The listing builds one solid part. Answer for the finished solid, in the listing's coordinates (mm). A direction names the side the tool comes from. Coordinates: 2 decimals unless noted, no trailing zeros. Loops run counter-clockwise (first coordinate to the right, second up) from the corner with the lowest first, then second, coordinate; pieces in that order, holes last. Notation, with made-up numbers: M -34.75,39 L -10.75,39 A20 ccw -10.75,78 Z; hole C -37.75,65.25 d1. An arc over 180 degrees is marked long. Answer as a JSON object with one key per item and string values. Group by question number.
1. A cutting plane is placed at A-A on y = 22. Give the vertices of the cut face in (x, z), and give its area (3 significant figures).
2. Given pin 1 (2 mm diameter, centred on x = 0, z = -4, fed in from +Y); pin 2 (1.5 mm diameter, centred on x = -2, z = -8.5, fed in from -Y), each flat-ended and moving along its own axis, determine where each tip first touches the part or whether it passes through.
3. For faces 1 (the face through (0, 19.05, -4)), 2 (the face through (-6.35, 13, -6)), determine the directions among +Z, -Z, +X, -X, +Y, -Y from which every point of the face is accessible in a straight line to the end or side of a thin tool.
4. Straight lines are drawn through the part: L1, parallel to Y at x = 0, z = -2.25; L2, parallel to Y at x = 0, z = -1.25; L3, parallel to Z at x = -0.75, y = 1.5. For each, find the intervals that lie inside material, in ascending order.
5. Determine the mould class of faces 3 (the face through (0, 0, -6.35)), 4 (the face through (3.804, 1.198, -3.131)), 5 (the face through (0, 25.4, -6)), 6 (the face through (0, 10, -12.7)) for opening direction Y: released by +Y, released by -Y, zero draft, split by the parting line, or undercut.
from build123d import *

# Parameters (mm, degrees)
SKETCH1_W           = 12.7
SKETCH1_H           = 19.05
SKETCH1_H_2         = 12.7
SKETCH1_R           = 3.9878
BOSS_EXTRUDE1_DEPTH = 12.7
FILLET1_SIZE        = 7.9756
CUT_EXTRUDE2_DEPTH  = 6.35
SKETCH1_3_R         = 3.9878
CUT_EXTRUDE3_DEPTH  = 6.35


with BuildPart() as part:
    # Sketch1 → Boss-Extrude1 (new body)
    # profile 1 of 3: a face of its own
    with BuildSketch(Plane.XY):
        with Locations((0, 15.875)):
            Rectangle(SKETCH1_W, SKETCH1_H)
    # profile 2 of 3: a face of its own
    with BuildSketch(Plane.XY):
        Rectangle(SKETCH1_W, SKETCH1_H_2)
        Circle(SKETCH1_R, mode=Mode.SUBTRACT)
    # profile 3 of 3: a face of its own
    with BuildSketch(Plane.XY):
        Circle(SKETCH1_R)
    extrude(amount=-BOSS_EXTRUDE1_DEPTH)

    # Fillet1
    # a fillet whose section is not a circle: 7.9756 mm, written as the material it takes off along each edge
    with BuildSketch(Plane(origin=(-6.35, -6.35, 19.939), x_dir=(1, 0, 0), z_dir=(0, 0, -1)), Plane(origin=(6.35, -6.35, 19.939), x_dir=(0, 1, 0), z_dir=(0, 0, -1))) as fillet1_piece_1:
        with BuildLine():
            add(Edge.make_bspline([(FILLET1_SIZE, 0), (FILLET1_SIZE * 0.831801948466, 0), (FILLET1_SIZE * 0.663603896932, 0), (FILLET1_SIZE * 0.292893218813, -FILLET1_SIZE * 0.0716919198361), (FILLET1_SIZE * 0.0716919198361, -FILLET1_SIZE * 0.292893218813), (0, -FILLET1_SIZE * 0.663603896932), (0, -FILLET1_SIZE * 0.831801948466), (0, -FILLET1_SIZE)], knots=[0, 0, 0, 0, 0, 0, 0.5, 0.5, 1, 1, 1, 1, 1, 1], degree=5))
            Line((0, -FILLET1_SIZE), (0, 0))
            Line((0, 0), (FILLET1_SIZE, 0))
        make_face()
    extrude(amount=52.578, mode=Mode.SUBTRACT)

    # Sketch3 → Cut-Extrude2 (cut)
    with BuildSketch(Plane(origin=(0, 25.4, 0), x_dir=(1, 0, 0), z_dir=(0, 1, 0))):
        with BuildLine():
            ThreePointArc((1.9939, 8.89), (1.409900211, 10.299900211), (0, 10.8839))
            Line((0, 10.8839), (0, 8.89))
            Line((0, 8.89), (1.9939, 8.89))
        make_face()
        with BuildLine():
            Line((0, 8.89), (0, 10.8839))
            ThreePointArc((0, 10.8839), (-1.409900211, 10.299900211), (-1.9939, 8.89))
            Line((-1.9939, 8.89), (0, 8.89))
        make_face()
        with BuildLine():
            Line((1.9939, 8.89), (0, 8.89))
            Line((0, 8.89), (0, 6.8961))
            ThreePointArc((0, 6.8961), (1.409900211, 7.480099789), (1.9939, 8.89))
        make_face()
        with BuildLine():
            Line((0, 6.8961), (0, 8.89))
            Line((0, 8.89), (-1.9939, 8.89))
            ThreePointArc((-1.9939, 8.89), (-1.409900211, 7.480099789), (0, 6.8961))
        make_face()
        with BuildLine():
            ThreePointArc((1.9939, 3.81), (1.409900211, 5.219900211), (0, 5.8039))
            Line((0, 5.8039), (0, 3.81))
            Line((0, 3.81), (1.9939, 3.81))
        make_face()
        with BuildLine():
            Line((0, 3.81), (0, 5.8039))
            ThreePointArc((0, 5.8039), (-1.409900211, 5.219900211), (-1.9939, 3.81))
            Line((-1.9939, 3.81), (0, 3.81))
        make_face()
        with BuildLine():
            ThreePointArc((0, 1.8161), (1.409900211, 2.400099789), (1.9939, 3.81))
            Line((1.9939, 3.81), (0, 3.81))
            Line((0, 3.81), (0, 1.8161))
        make_face()
        with BuildLine():
            Line((0, 3.81), (-1.9939, 3.81))
            ThreePointArc((-1.9939, 3.81), (-1.409900211, 2.400099789), (0, 1.8161))
            Line((0, 1.8161), (0, 3.81))
        make_face()
    extrude(amount=-CUT_EXTRUDE2_DEPTH, mode=Mode.SUBTRACT)

    # Sketch1<3> → Cut-Extrude3 (cut)
    with BuildSketch(Plane.XY):
        Circle(SKETCH1_3_R)
    extrude(amount=-CUT_EXTRUDE3_DEPTH, mode=Mode.SUBTRACT)


solid = part.part
From the geometry:
{
 "1": {"outline": "M -6.35,-12.7 L 6.35,-12.7 L 6.35,0 L -6.35,0 Z; hole C 0,-8.89 d3.99; hole C 0,-3.81 d3.99", "area": "136 mm²"},
 "2": {"pin 1": "stops at y = 19.05", "pin 2": "stops at y = -6.17"},
 "3": {"face 1": "+Y", "face 2": "+Z, -Z, -X, +Y, -Y"},
 "4": {"L1": "y = -6.31 to -3.99, 3.99 to 19.05", "L2": "y = -6.31 to -3.99, 3.99 to 25.4", "L3": "z = -12.7 to -6.35"},
 "5": {"face 3": "undercut", "face 4": "undercut", "face 5": "released by +Y", "face 6": "zero draft"}
}
